```python
from build123d import *

# Parameters (mm, degrees)
F0_R     = 5.25
F1_DEPTH = 0.95
F3_DEPTH = 3.25
F4_R     = 2.09999
F5_R     = 1.15
F6_DEPTH = 25


# Not quite as in the source:
# - a fillet or chamfer is up to 0.001 mm smaller than in the source, because OpenCascade refuses the exact size


with BuildPart() as f1:
    # F0 (on Top) → F1 (new body)
    with BuildSketch(Plane.XY):
        with BuildLine():
            Line((20.596680348, 5.4), (24.5, 5.4))
            Line((24.5, 5.4), (24.5, 9.6))
            Line((24.5, 9.6), (20.596680348, 9.6))
            ThreePointArc((20.596680348, 9.6), (18.5774207214, 9.8769403602), (16.7072849584, 10.6873091839))
            Line((16.7072849584, 10.6873091839), (11.3893953897, 13.9126908161))
            ThreePointArc((11.3893953897, 13.9126908161), (9.5192596266, 14.7230596398), (7.5, 15))
            ThreePointArc((7.5, 15), (2.1966991411, 12.8033008589), (0, 7.5))
            ThreePointArc((0, 7.5), (2.1966991411, 2.1966991411), (7.5, 0))
            ThreePointArc((7.5, 0), (9.5192596266, 0.2769403602), (11.3893953897, 1.0873091839))
            Line((11.3893953897, 1.0873091839), (16.7072849584, 4.3126908161))
            ThreePointArc((16.7072849584, 4.3126908161), (18.5774207214, 5.1230596398), (20.596680348, 5.4))
        make_face()
        with Locations((7.5, 7.5)):
            Circle(F0_R, mode=Mode.SUBTRACT)
    extrude(amount=F1_DEPTH)

    # F2 (on face) → F3 (join)
    with BuildSketch(Plane.XY.offset(0.95)):
        Polygon((24.5, 5.4), (24.5, 9.6), (20.596680348, 9.6), (20, 9.6), (20, 5.4), (20.596680348, 5.4), align=None)
    extrude(amount=F3_DEPTH)

    # F4 (radius 2.1 in the source; OpenCascade refuses exactly that, so slightly less here)
    f4_edges = [f1.edges().sort_by_distance(p)[0] for p in [
        (22.25, 9.6, 4.2),
        (22.25, 5.4, 4.2),
    ]]
    fillet(f4_edges, radius=F4_R)

    # F5 (on face) → F6 (cut)
    with BuildSketch(Plane.YZ.offset(24.5)):
        with Locations((7.5, 2.1)):
            Circle(F5_R)
    extrude(amount=-F6_DEPTH, mode=Mode.SUBTRACT)


solid = f1.part
```
Geometry: final body of the model. Coordinates: model frame, mm. A direction names the side the tool comes from. Round coordinates to 2 decimals unless told otherwise and drop trailing zeros. Write each loop counter-clockwise with the first axis right and the second up, starting at its lowest first coordinate (ties: lowest second). Pieces come first, ordered by that corner, then holes.
Item 1: Set-up query: faces 5 (the face through (20, 7.5, 3.6)), 6 (the face through (14.086, 12.277, 0.468)). Return all of +Z, -Z, +X, -X, +Y, -Y with unobstructed straight access to the full face (end or side cutting, diameter ignored); none if empty.
Item 2: Pin query (flat end, axial travel): P1, Ø8, axis at x = 7.5, y = 6.5, coming from the +Z side; P2, Ø1, axis at y = 8.5, z = 2.5, coming from the -X side; P3, Ø1.1, axis at x = 22.5, z = 1.5, coming from the -Y side; P4, Ø1.5, axis at x = 14, z = 1, coming from the +Y side. Return the tip coordinate at first contact, or that it passes through.
Item 3: Section query A-A (z = 2.65). Return loops of the section in (x, y).
Item 4: Material intervals for L1, parallel to Y at x = 7.5, z = 0.4; L2, parallel to X at y = 7.5, z = 0.6; L3, parallel to Z at x = 23.35, y = 7.5, sorted ascending.
Item 5: Mould query, pull axis Y, two halves, no side actions, for faces 1 (the face through (22, 9.6, 1)), 2 (the face through (12, 11, 0.95)), 3 (the face through (10.32, 11.93, 0.47)), 4 (the face through (22.282, 8.597, 2.445)). Classes: +Y half, -Y half, draft (parallel to the pull), parting line (faces both ways), or undercut.
Item 6: Section query D-D (y = 13). Return loops of the section in (x, z), plus the area to 3 significant figures.
Item 7: Section query B-B (x = 7.75). Return loops of the section in (y, z).
Item 8: Section query C-C (y = 7). Return loops of the section in (x, z).
Completed:
1. face 5: +Z, -X, +Y, -Y
1. face 6: +Z, -Z, +X, +Y
2. P1: passes through
2. P2: stops at x = 20
2. P3: stops at y = 5.4
2. P4: stops at y = 12.78
3. outline: (20, 5.47) - (24.5, 5.47) - (24.5, 6.49) - (20, 6.49) - close; (20, 8.51) - (24.5, 8.51) - (24.5, 9.53) - (20, 9.53) - close
4. L1: y = 0 to 2.25, 12.75 to 15
4. L2: x = 0 to 2.25, 12.75 to 24.5
4. L3: z = 0 to 0.95, 3.25 to 4.2
5. face 1: +Y half
5. face 2: draft
5. face 3: undercut
5. face 4: undercut
6. outline: (2.4, 0) - (12.89, 0) - (12.89, 0.95) - (2.4, 0.95) - close
6. area: 9.97 mm2
7. outline: (0, 0) - (2.26, 0) - (2.26, 0.95) - (0, 0.95) - close; (12.74, 0) - (15, 0) - (15, 0.95) - (12.74, 0.95) - close
8. outline: (0.02, 0) - (2.27, 0) - (2.27, 0.95) - (0.02, 0.95) - close; (12.73, 0) - (24.5, 0) - (24.5, 1.06) - (20, 1.06) - (20, 0.95) - (12.73, 0.95) - close; (20, 3.14) - (24.5, 3.14) - (24.5, 4.14) - (20, 4.14) - close
